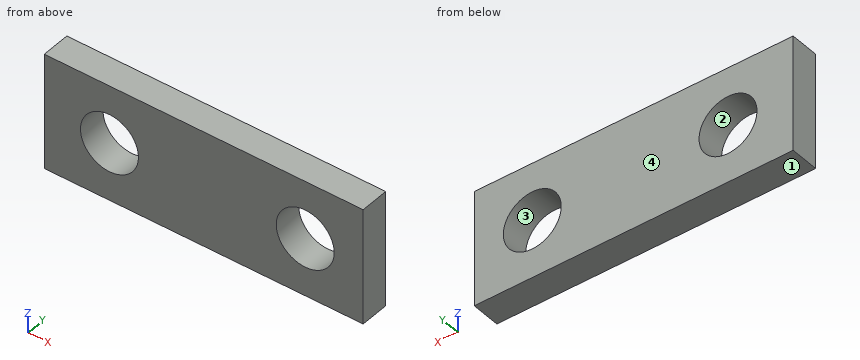
Autodesk Fusion 360 part; units mm, degrees
sketch "Sketch1" plane through (0, 0, 0) normal (0, 1, 0) x (1, 0, 0)
  line L0 (0, 0) -> (69.85, 0)
  line L1 (69.85, 0) -> (69.85, -25.4)
  line L2 (69.85, -25.4) -> (0, -25.4)
  line L3 (0, -25.4) -> (0, 0)
  circle A0 centre (57.15, -12.7) radius 6.35
  line L4 (34.925, -25.4) -> (34.925, 0) construction
  circle A1 centre (14.2748, -12.7) radius 6.35
  dimension "d1" = 69.85
  dimension "d2" = 25.4
  dimension "d3" = 12.7
  dimension "d4" = 12.7
  dimension "d5" = 12.7
  dimension "d6" = 14.2748
extrude "Extrude1" add sketch "Sketch1" along normal blind 6.35
Input: part model. Units: mm. Frame: model coordinates. Face numbers are marked on the shaded views. Give positions to 0.01 mm unless a question says otherwise; leave off trailing zeros. Order: outer loops, then holes, each group sorted by start corner. A loop starts at its lowest first (then second) coordinate and runs counter-clockwise, first axis right, second up. Notation, with made-up numbers: (10, 22) - (34, 22) arc R11 ccw to (34, 43) - close; hole circle Ø9 at (-11.5, -12). An arc over 180 degrees is marked (long way). Answer as a JSON object with one key per item and string values. Group by question number.
Q1. Cut plane A-A, the plane x = 57.15. Output: boundary loops of the cut face in (y, z), then the cut area to 3 significant figures.
Q2. First-contact query: pin 1 Ø12 at (x, z) = (19.5, 5) entering from -Y. Flat tip, straight axial feed; report the tip coordinate or a pass-through.
Q3. Cut plane C-C, the plane y = 4.25. Output: boundary loops of the cut face in (x, z), then the cut area to 3 significant figures.
Q4. Mould query, pull axis Z, two halves, no side actions, for the marked faces 1, 2, 3 and 4. Classes: pulls with the +Z half, pulls with the -Z half, needs draft (parallel to the pull), parting line crosses it, or undercut.
Q5. Cut plane B-B, the plane z = 12.7. Output: boundary loops of the cut face in (x, y), then the cut area to 3 significant figures.
Q6. Line query: probe 1 along X at (y, z) = (3.5, 12.7); probe 2 along Z at (x, y) = (57.15, 4.25); probe 3 along X at (y, z) = (2, 17.25). Output: solid intervals per line, ascending.
Q7. Cut plane D-D, the plane x = 9. Output: boundary loops of the cut face in (y, z), then the cut area to 3 significant figures.
Results:
{
 "1": {"outline": "(0, 0) - (6.35, 0) - (6.35, 6.35) - (0, 6.35) - close; (0, 19.05) - (6.35, 19.05) - (6.35, 25.4) - (0, 25.4) - close", "area": "80.6 mm^2"},
 "2": {"pin 1": "y = 0"},
 "3": {"outline": "(0, 0) - (69.85, 0) - (69.85, 25.4) - (0, 25.4) - close; hole circle Ø12.7 at (14.27, 12.7); hole circle Ø12.7 at (57.15, 12.7)", "area": "1,520 mm^2"},
 "4": {"face 1": "pulls with the -Z half", "face 2": "undercut", "face 3": "undercut", "face 4": "needs draft"},
 "5": {"outline": "(0, 0) - (7.92, 0) - (7.92, 6.35) - (0, 6.35) - close; (20.62, 0) - (50.8, 0) - (50.8, 6.35) - (20.62, 6.35) - close; (63.5, 0) - (69.85, 0) - (69.85, 6.35) - (63.5, 6.35) - close", "area": "282 mm^2"},
 "6": {"probe 1": "0 to 7.92, 20.62 to 50.8, 63.5 to 69.85", "probe 2": "0 to 6.35, 19.05 to 25.4", "probe 3": "0 to 9.85, 18.7 to 52.72, 61.58 to 69.85"},
 "7": {"outline": "(0, 0) - (6.35, 0) - (6.35, 9.16) - (0, 9.16) - close; (0, 16.24) - (6.35, 16.24) - (6.35, 25.4) - (0, 25.4) - close", "area": "116 mm^2"}
}
